```python
from build123d import *

# Parameters (mm, degrees)
F2_SIZE = 0.09999


# Not quite as in the source:
# - a fillet or chamfer is up to 0.001 mm smaller than in the source, because OpenCascade refuses the exact size


with BuildPart() as f1:
    # F0 (on Right) → F1 (revolve)
    with BuildSketch(Plane.YZ):
        Polygon((6.425, 3.3), (6.925, 2.8), (6.925, 3.3), align=None)
        with BuildLine():
            ThreePointArc((7.5617104388, 2.8), (8.3591026496, 4.0638625595), (9.425, 5.1112620751))
            Line((9.425, 5.1112620751), (9.425, 5.9))
            Line((9.425, 5.9), (-18.075, 5.9))
            Line((-18.075, 5.9), (-18.075, 3.4))
            Line((-18.075, 3.4), (-7.075, 3.4))
            Line((-7.075, 3.4), (-7.075, 3.3))
            Line((-7.075, 3.3), (-6.425, 3.3))
            Line((-6.425, 3.3), (6.425, 3.3))
            Line((6.425, 3.3), (6.925, 3.3))
            Line((6.925, 3.3), (6.925, 2.8))
            Line((6.925, 2.8), (7.5617104388, 2.8))
        make_face()
    revolve(axis=Axis((0, 1.2040399015, 0), (0, 1, 0)))

    # F2 (size 0.1 in the source; OpenCascade refuses exactly that, so slightly less here)
    f2_edges = [f1.edges().sort_by_distance(p)[0] for p in [
        (0, -7.075, -3.4),
    ]]
    chamfer(f2_edges, length=F2_SIZE)


solid = f1.part
```
Work out the finished part from the listing and answer in its coordinate system (mm). A direction names the side the tool comes from. Give positions to 0.01 mm unless a question says otherwise; leave off trailing zeros. Loops run counter-clockwise (first coordinate to the right, second up) from the corner with the lowest first, then second, coordinate; pieces in that order, holes last. Notation, with made-up numbers: (5.5, 20) -> (13.5, 20) arc R14 ccw to (13.5, 29) -> close; hole circle Ø10 at (60.5, 67.25). An arc over 180 degrees is marked (long way). Put each result on its own line as item: value. Start each with the question number.
Item 1: Which of the six approach directions +Z, -Z, +X, -X, +Y, -Y give full straight-line access (tool end or side, diameter ignored) to faces 1 (the face through (5, 9.425, 2)), 2 (the face through (-3.32, -12.55, -0.74))?
Item 2: The part is cut by section C-C (y = -11). Give the vertices of the cut face in (x, z), then the cut area to 3 significant figures.
Item 3: Each of these flat-tipped pins is pushed along its axis until it touches: P1, Ø3.5, axis at x = 0, z = 0, coming from the -Y side; P2, Ø6, axis at x = 0, z = 0, coming from the -Y side (3 decimals); P3, Ø3, axis at x = 3.5, y = 3.5, coming from the -Z side; P4, Ø5, axis at y = -7.5, z = 4.5, coming from the -X side. Where does it stop, or does it pass through?
Item 4: The mould has two halves that part along Z. Classify faces 3 (the face through (2.23, -0.23, -2.43)), 4 (the face through (0.259, -4.518, -5.894)), 5 (the face through (0.1, 7.2, -2.8)), 6 (the face through (-3, -18.075, 3)): released by +Z, released by -Z, zero draft, split by the parting line, or undercut.
Item 5: The part is cut by section D-D (y = 4). Give the vertices of the cut face in (x, z).
Item 6: Find the intervals of material crossed by L1, parallel to X at y = -14.25, z = 0; L2, parallel to X at y = 1.75, z = 0; L3, parallel to Z at x = 3, y = -11.25, in increasing order. Write a range as [from, to].
Answers below:
1. face 1: +Z, -Z, +X, -X, +Y
1. face 2: -Y
2. outline: circle Ø11.8 at (0, 0); hole circle Ø6.8 at (0, 0)
2. area: 73.0 mm2
3. P1: through
3. P2: y = 6.725
3. P3: z = -5.55
3. P4: x = -5.55
4. face 3: undercut
4. face 4: split by the parting line
4. face 5: undercut
4. face 6: zero draft
5. outline: circle Ø11.8 at (0, 0); hole circle Ø6.6 at (0, 0)
6. L1: [-5.9, -3.4], [3.4, 5.9]
6. L2: [-5.9, -3.3], [3.3, 5.9]
6. L3: [-5.08, -1.6], [1.6, 5.08]
